```python
from build123d import *

# Parameters (mm, degrees)
F1_DEPTH = 6
F2_R     = 0.99999


# Not quite as in the source:
# - a fillet or chamfer is up to 0.001 mm smaller than in the source, because OpenCascade refuses the exact size


with BuildPart() as f1:
    # F0 (on Top) → F1 (new body)
    with BuildSketch(Plane.XY):
        with BuildLine():
            Line((-79.3681601882, 18.7270958871), (-79.3681601882, 21.703983524))
            Line((-79.3681601882, 21.703983524), (-73.7681601882, 21.703983524))
            Line((-73.7681601882, 21.703983524), (-73.7681601882, 20.203983524))
            Line((-73.7681601882, 20.203983524), (-77.3441610362, 17.968982994))
            ThreePointArc((-77.3441610362, 17.968982994), (-77.566357164, 17.6574135954), (-77.5031607182, 17.279984372))
            Line((-77.5031607182, 17.279984372), (-76.9731617782, 16.431986068))
            ThreePointArc((-76.9731617782, 16.431986068), (-76.6615923795, 16.2097899402), (-76.2841631562, 16.272986386))
            Line((-76.2841631562, 16.272986386), (-72.7081623082, 18.507986916))
            ThreePointArc((-72.7081623082, 18.507986916), (-72.0188752257, 19.2344464592), (-71.7681601882, 20.203983524))
            Line((-71.7681601882, 20.203983524), (-71.7681601882, 21.703983524))
            ThreePointArc((-71.7681601882, 21.703983524), (-72.3539466258, 23.1181970864), (-73.7681601882, 23.703983524))
            Line((-73.7681601882, 23.703983524), (-79.3681601882, 23.703983524))
            ThreePointArc((-79.3681601882, 23.703983524), (-80.7823737506, 23.1181970864), (-81.3681601882, 21.703983524))
            Line((-81.3681601882, 21.703983524), (-81.3681601882, 20.3047729959))
            ThreePointArc((-81.3681601882, 20.3047729959), (-82.5569903042, 16.8343446369), (-79.3681601882, 15.0209079738))
            Line((-79.3681601882, 15.0209079738), (-79.3681601882, 16.9770958871))
            Line((-79.3681601882, 16.9770958871), (-79.8681601882, 16.9770958871))
            ThreePointArc((-79.8681601882, 16.9770958871), (-80.7431601882, 17.8520958871), (-79.8681601882, 18.7270958871))
            Line((-79.8681601882, 18.7270958871), (-79.3681601882, 18.7270958871))
        make_face()
    extrude(amount=F1_DEPTH)

    # F2 (radius 1 in the source; OpenCascade refuses exactly that, so slightly less here)
    f2_edges = [f1.edges().sort_by_distance(p)[0] for p in [
        (-79.36816, 15.020908, 3),
        (-79.36816, 18.727096, 3),
        (-79.36816, 16.977096, 3),
    ]]
    fillet(f2_edges, radius=F2_R)


solid = f1.part
```
Can you work these out from the model? Positions are in its coordinate system, mm. A direction names the side the tool comes from. Give positions to 0.01 mm unless a question says otherwise; leave off trailing zeros. Loops run counter-clockwise (first coordinate to the right, second up) from the corner with the lowest first, then second, coordinate; pieces in that order, holes last. Notation, with made-up numbers: M 41,86.5 L 96,86.5 A17 cw 96,94.5 Z; hole C 36,31.25 d4. An arc over 180 degrees is marked long. Answer in a Markdown table with one row per item.
1. Suppose I cut it at B-B on x = -74. Write out the boundary of the cut face in (y, z), plus the area to 3 significant figures.
Taken from the geometry:
| item | result |
|---|---|
| outline | M 17.7,0 L 20.06,0 L 20.06,6 L 17.7,6 Z; M 21.7,0 L 23.7,0 L 23.7,6 L 21.7,6 Z |
| area | 26.2 mm² |
2. Which directions (+Z, -Z, +X, -X, +Y, -Y) give clear straight access to the entire face, cutting with the end or side of a thin tool? Please do faces 4 (the flat face through (-79.368, 21, 3)), 5 (the flat face through (-73.768, 21, 3)), 6 (the flat face through (-81.368, 21, 3)).
Taken from the geometry:
| item | result |
|---|---|
| face 4 | +Z, -Z, -Y |
| face 5 | +Z, -Z |
| face 6 | +Z, -Z, -X, +Y |
3. Suppose I cut it at A-A on y = 20.75. Write out the boundary of the cut face in (x, z), plus the area to 3 significant figures.
Taken from the geometry:
| item | result |
|---|---|
| outline | M -81.37,0 L -79.37,0 L -79.37,6 L -81.37,6 Z; M -73.77,0 L -71.77,0 L -71.77,6 L -73.77,6 Z |
| area | 24.0 mm² |
4. For pin 1 Ø1.6 at (y, z) = (21, 4.5) entering from -X; pin 2 Ø1 at (x, z) = (-73.5, 4) entering from -Y; pin 3 Ø3 at (x, z) = (-77, 3.5) entering from -Y, each with a flat end and sliding along its axis, tell me the tip position at first contact or that it passes through.
Taken from the geometry:
| item | result |
|---|---|
| pin 1 | stops at x = -81.53 |
| pin 2 | stops at y = 17.7 |
| pin 3 | stops at y = 16.2 |
5. Suppose I cut it at C-C on x = -78.5. Write out the boundary of the cut face in (y, z), plus the area to 3 significant figures.
Taken from the geometry:
| item | result |
|---|---|
| outline | M 21.7,0 L 23.7,0 L 23.7,6 L 21.7,6 Z |
| area | 12.0 mm² |
6. Suppose I cut it at D-D on y = 22. Write out the boundary of the cut face in (x, z), plus the area to 3 significant figures.
Taken from the geometry:
| item | result |
|---|---|
| outline | M -81.35,0 L -71.79,0 L -71.79,6 L -81.35,6 Z |
| area | 57.3 mm² |
7. Thinking about a two-plate mould opening in X: for faces 1 (the flat face through (-76, 18, 0)), 2 (the flat face through (-77, 21.704, 3)), 3 (the cylindrical face through (-79.773, 15.241, 3.042)), which applies, released by +X, released by -X, zero draft, split by the parting line, or undercut?
Taken from the geometry:
| item | result |
|---|---|
| face 1 | zero draft |
| face 2 | undercut |
| face 3 | split by the parting line |
8. If I drill on line 1 along X through (y, z) = (21, 0.25); line 2 along X through (y, z) = (21.75, 2); line 3 along Y through (x, z) = (-79, 2.25), over which ranges is the centre line in solid material (lowest first)?
Taken from the geometry:
| item | result |
|---|---|
| line 1 | x = -81.37 to -79.37, -73.77 to -71.77 |
| line 2 | x = -81.37 to -71.77 |
| line 3 | y = 21.7 to 23.7 |
